Model file for the job. Use its own axes, mm. A direction names the side the tool comes from. Give positions to 0.01 mm unless a question says otherwise; leave off trailing zeros. Order: outer loops, then holes, each group sorted by start corner. A loop starts at its lowest first (then second) coordinate and runs counter-clockwise, first axis right, second up. Notation, with made-up numbers: (-15.75, 76.5) - (29.25, 76.5) arc R14 ccw to (29.25, 86.5) - close; hole circle Ø2 at (-13, 87). An arc over 180 degrees is marked (long way). Use CSV: the item, a comma, the result in double quotes. Start each with the question number.
(1) Band-saw the part on B-B, the plane y = -11. Give the cut face in (x, z), then the cut area to 3 significant figures.
(2) Tool access for faces 1 (the flat face through (0, 15, 2)), 2 (the flat face through (-3.43, 9.616, 1.972)): list every direction of +Z, -Z, +X, -X, +Y, -Y with a clear straight run to the whole face (end or side of a thin tool).
(3) Band-saw the part on A-A, the plane z = 3.3. Give the cut face in (x, y), then the cut area to 3 significant figures.
(4) Probe L1, parallel to Y at x = -1.25, z = 2.8; L2, parallel to Y at x = -5, z = 0.95; L3, parallel to X at y = -12, z = 0.85. List the from-to ranges inside material, lowest first.
(5) Pull direction Y, two halves, no side cores. Call faces 3 (the flat face through (-3.43, -13.284, 1.972)), 4 (the flat face through (-5, -16.45, 2)), 5 (the flat face through (-5, 16.45, 2)), 6 (the flat face through (-10, 0, 2)): +Y half, -Y half, draft (parallel to the pull), parting line (faces both ways), or undercut.
(6) Drop a flat-ended pin along its axis: pin 1 Ø1 at (y, z) = (10.5, 1.5) entering from +X. Give the stop position or say it passes through.
from build123d import *
from OCP.BRepFilletAPI import BRepFilletAPI_MakeChamfer

# Parameters (mm, degrees)
BOSS_EXTRUDE1_DEPTH = 4
CHAMFER1_SIZE       = 0.7
CHAMFER1_SIZE2      = 0.736453843


with BuildPart() as part:
    # Sketch1 → Boss-Extrude1 (new body)
    with BuildSketch(Plane.XY):
        Polygon((-10, 0), (0, 0), (0, 9.45), (-6.2, 9.75), (-6.2, 13.15), (0, 13.45), (0, 16.45), (-10, 16.45), align=None)
        Polygon((-6.2, -9.75), (0, -9.45), (0, 0), (-10, 0), (-10, -16.45), (0, -16.45), (0, -13.45), (-6.2, -13.15), align=None)
    extrude(amount=BOSS_EXTRUDE1_DEPTH)

    # Chamfer1: one chamfer whose edges measure the first distance from different faces: ONE call of the kernel's chamfer builder (chamfer() names one face for all edges)
    chamfer1_edges_1 = [part.edges().sort_by_distance(p)[0] for p in [
        (0, 13.45, 2),
    ]]
    chamfer1_side_1 = [part.faces().sort_by_distance(p)[0] for p in [
        (-3.1, 13.3, 2),
    ]]
    chamfer1_edges_2 = [part.edges().sort_by_distance(p)[0] for p in [
        (0, 9.45, 2),
    ]]
    chamfer1_side_2 = [part.faces().sort_by_distance(p)[0] for p in [
        (0, 0, 2),
    ]]
    chamfer1_edges_3 = [part.edges().sort_by_distance(p)[0] for p in [
        (0, -9.45, 2),
    ]]
    chamfer1_side_3 = [part.faces().sort_by_distance(p)[0] for p in [
        (-3.1, -9.6, 2),
    ]]
    chamfer1_edges_4 = [part.edges().sort_by_distance(p)[0] for p in [
        (0, -13.45, 2),
    ]]
    chamfer1_side_4 = [part.faces().sort_by_distance(p)[0] for p in [
        (0, -14.95, 2),
    ]]
    chamfer1 = BRepFilletAPI_MakeChamfer(part.part.solid().wrapped)
    for e in chamfer1_edges_1:
        chamfer1.Add(CHAMFER1_SIZE, CHAMFER1_SIZE2, e.wrapped, chamfer1_side_1[0].wrapped)  # the first distance lies on this face
    for e in chamfer1_edges_2:
        chamfer1.Add(CHAMFER1_SIZE, CHAMFER1_SIZE2, e.wrapped, chamfer1_side_2[0].wrapped)  # the first distance lies on this face
    for e in chamfer1_edges_3:
        chamfer1.Add(CHAMFER1_SIZE, CHAMFER1_SIZE2, e.wrapped, chamfer1_side_3[0].wrapped)  # the first distance lies on this face
    for e in chamfer1_edges_4:
        chamfer1.Add(CHAMFER1_SIZE, CHAMFER1_SIZE2, e.wrapped, chamfer1_side_4[0].wrapped)  # the first distance lies on this face
    add(Compound.cast(chamfer1.Shape()), mode=Mode.REPLACE)


solid = part.part
Answer block:
1,outline,"(-10, 0) - (-6.2, 0) - (-6.2, 4) - (-10, 4) - close"
1,area,"15.2 mm2"
2,face 1,"+Z, -Z, +X, +Y, -Y"
2,face 2,"+Z, -Z, +X"
3,outline,"(-10, -16.45) - (0, -16.45) - (0, -14.15) - (-0.74, -13.41) - (-6.2, -13.15) - (-6.2, -9.75) - (-0.7, -9.48) - (0, -8.71) - (0, 8.75) - (-0.74, 9.49) - (-6.2, 9.75) - (-6.2, 13.15) - (-0.7, 13.42) - (0, 14.19) - (0, 16.45) - (-10, 16.45) - close"
3,area,"282 mm2"
4,L1,"y = -16.45 to -13.39, -9.51 to 9.51, 13.39 to 16.45"
4,L2,"y = -16.45 to -13.21, -9.69 to 9.69, 13.21 to 16.45"
4,L3,"x = -10 to -6.2"
5,face 3,"undercut"
5,face 4,"-Y half"
5,face 5,"+Y half"
5,face 6,"draft"
6,pin 1,"stops at x = -6.2"
